Can you work these out from the model? Positions are in its coordinate system, mm. A direction names the side the tool comes from. Round coordinates to 2 decimals unless told otherwise and drop trailing zeros. Write each loop counter-clockwise with the first axis right and the second up, starting at its lowest first coordinate (ties: lowest second). Pieces come first, ordered by that corner, then holes. Notation, with made-up numbers: (43.25, 87) -> (71.25, 87) arc R35 cw to (71.25, 120) -> close; hole circle Ø8 at (58, -37.75). An arc over 180 degrees is marked (long way). Write item = value, one per line. Start each with the question number.
1) Imagine slicing it at A-A, the plane z = -21. Please give me the cut outline in (x, y), then the cut area to 3 significant figures.
2) Imagine slicing it at C-C, the plane x = -27. Please give me the cut outline in (y, z), then the cut area to 3 significant figures.
3) Imagine slicing it at B-B, the plane y = -12. Please give me the cut outline in (x, z).
4) For faces 1 (the face through (-23, 5.08, -13)), 2 (the face through (-23, -5.08, -13)), 3 (the face through (-16, 309.88, -10)), which set-ups out of +Z, -Z, +X, -X, +Y, -Y let a thin tool reach every point of the face, with its end or its side?
5) If I drill on line 1 (X direction, y = 257, z = -8.5); line 2 (Y direction, x = -7.5, z = -4); line 3 (X direction, y = 257.5, z = -10.25), over which ranges is the centre line in solid material (lowest first)?
6) I'm going to push flat-ended pins straight in: pin 1 (4 mm diameter, centred on y = 157, z = -9.5, fed in from -X); pin 2 (6 mm diameter, centred on y = 74.5, z = -7.5, fed in from +X); pin 3 (4 mm diameter, centred on x = -13.5, y = 41, fed in from -Z). Where does each tip first touch, or does it pass through?
7) Imagine slicing it at D-D, the plane y = 125. Please give me the cut outline in (x, z).
Autodesk Inventor part; units mm, degrees
ref_plane "YZ Plane" through (0, 0, 0) normal (1, 0, 0) x (0, 1, 0)
ref_plane "XZ Plane" through (0, 0, 0) normal (0, 1, 0) x (-1, 0, 0)
ref_plane "XY Plane" through (0, 0, 0) normal (0, 0, 1) x (1, 0, 0)
sketch "Base" plane through (0, 0, 0) normal (0, 1, 0) x (-1, 0, 0)
  circle A0 centre (16.3612, -10.3188) radius 6.35
  line L0 (-4.6434, -3.9692) -> (-4.6434, -16.6683)
  point P0 (0, 0)
  point P1 (16.4327, -3.9692)
extrude "ForwardFeature" add sketch "Base" along normal blind 309.88 draft -0.5
sketch "Sketch2" plane through (-16.3612, 0, -10.3188) normal (0, -1, 0) x (1, 0, 0)
  circle A0 centre (0, 0) radius 6.35
  point P0 (16.3612, 10.3188)
extrude "BackFeature" add sketch "Sketch2" along normal blind 88.9
sketch "Sketch3" plane through (0, 0, 0) normal (0, 1, 0) x (-1, 0, 0)
  circle A0 centre (16.3612, -10.3188) radius 14.2875
  line L0 (-4.6434, -24.6063) -> (-4.6434, 3.9686)
  point P0 (0, 0)
extrude "CollarFeature" add sketch "Sketch3" along normal mid plane 10.16
properties part number "DrumstickBoundingBox"
Reported:
q1.outline = (-25.85, -5.08) -> (-6.87, -5.08) -> (-6.87, 5.08) -> (-25.85, 5.08) -> close
q1.area = 193 mm²
q2.outline = (-5.08, -19.86) -> (5.08, -19.86) -> (5.08, -0.78) -> (-5.08, -0.78) -> close
q2.area = 194 mm²
q3.outline = circle Ø12.7 at (-16.36, -10.32)
q4.face_1 = +Y
q4.face_2 = -Y
q4.face_3 = +Z, -Z, +X, -X, +Y
q5.line_1 = -20.04 to -12.68
q5.line_2 = -5.08 to 5.08
q5.line_3 = -20.46 to -12.26
q6.pin_1 = -21.36
q6.pin_2 = -10.65
q6.pin_3 = -16.25
q7.outline = circle Ø10.52 at (-16.36, -10.32)
